Read the model definition and answer for the solid it produces. Units are mm, in the model's axes. A direction names the side the tool comes from. Coordinates: 2 decimals unless noted, no trailing zeros. Loops run counter-clockwise (first coordinate to the right, second up) from the corner with the lowest first, then second, coordinate; pieces in that order, holes last. Notation, with made-up numbers: (-38.75, -12.75) - (-31.75, -12.75) arc R24 ccw to (-31.75, 9.25) - close; hole circle Ø9 at (3.25, 38). An arc over 180 degrees is marked (long way). Use one line per item in the form item = value. Start each with the question number.
1) A cutting plane is placed at B-B (z = -8). Give the vertices of the cut face in (x, y) (3 decimals), and give its area (3 significant figures).
2) A cutting plane is placed at C-C (z = -14.5). Give the vertices of the cut face in (x, y) (3 decimals), and give its area (3 significant figures).
3) A cutting plane is placed at A-A (y = 10.85). Give the vertices of the cut face in (x, z) (3 decimals), and give its area (3 significant figures).
4) Which of the six approach directions +Z, -Z, +X, -X, +Y, -Y give full straight-line access (tool end or side, diameter ignored) to faces 4 (the face through (135, 12, -5.08)), 5 (the face through (135, 3, -19.05)), 6 (the face through (135, 47.117, 10))?
5) A cutting plane is placed at D-D (z = 8). Give the vertices of the cut face in (x, y) (3 decimals), and give its area (3 significant figures).
6) Consider line 1 (Y direction, x = 135.15, z = 10.5); line 2 (Y direction, x = 135, z = -8); line 3 (Y direction, x = 133.9, z = 23.5). Determine where each line is inside the solid, lowest interval first.
7) Each of these flat-tipped pins is pushed along its axis until it touches: P1, Ø1, axis at x = 134.5, y = 84.5, coming from the -Z side; P2, Ø1.6, axis at x = 135.5, y = 18, coming from the +Z side; P3, Ø1, axis at x = 135.5, z = -26.5, coming from the -Y side; P4, Ø5, axis at y = 10.85, z = 14.5, coming from the +X side (3 decimals). Where does it stop, or does it pass through?
8) The mould has two halves that part along Z. Classify faces 1 (the face through (134.96, 64.337, 8.195)), 2 (the face through (135, 43.942, -4)), 3 (the face through (135, 81, -25.4)): released by +Z, released by -Z, zero draft, split by the parting line, or undercut.
from build123d import *

# Parameters (mm, degrees)
SKETCH1_W              = 273.05
SKETCH1_H              = 139.7
BOSS_EXTRUDE1_DEPTH    = 6.35
SKETCH2_W              = 273.05
SKETCH2_H              = 139.7
SKETCH2_W_2            = 266.7
SKETCH2_H_2            = 133.35
BOSS_EXTRUDE2_DEPTH    = 298.45
SKETCH3_W              = 6.35
SKETCH3_H              = 16.933333333
SKETCH3_H_2            = 16.933333334
DOOR_SLOT_DEPTH        = 12.7
DOOR_GUIDE_HOLES_REACH = 362.806
SKETCH4_W              = 6.35
SKETCH4_H              = 15.875
LEVER_HOLES_W          = 9.652
LEVER_HOLES_H          = 6.35
LEVER_HOLES_W_2        = 6.35
CUT_EXTRUDE1_DEPTH     = 363.019620497
CUT_EXTRUDE3_REACH     = 417.137
SKETCH8_R              = 3.175
SKETCH16_W             = 329.651778096
SKETCH16_H             = 315.233565403
CUT_EXTRUDE10_DEPTH    = 363.019620497
LEFT_RIGHT_W           = 9.525
LEFT_RIGHT_H           = 6.35
LEFT_RIGHT_W_2         = 12.7
LEFT_RIGHT_W_3         = 3.175
LEFT_RIGHT_H_2         = 12.7
CUT_EXTRUDE11_DEPTH    = 416.136561869
SKETCH17_W             = 23
SKETCH17_H             = 20.0007988
SKETCH17_W_2           = 10.16
SKETCH17_H_2           = 5.89
SKETCH17_R             = 1.5
CUT_EXTRUDE12_DEPTH    = 313.717353412
CUT_EXTRUDE13_DEPTH    = 313.717353412
CUT_EXTRUDE14_DEPTH    = 106.589636092


with BuildPart() as part:
    # Sketch1 → Boss-Extrude1 (new body)
    with BuildSketch(Plane(origin=(0, 0, 0), x_dir=(1, 0, 0), z_dir=(0, 1, 0))):
        Rectangle(SKETCH1_W, SKETCH1_H)
    extrude(amount=BOSS_EXTRUDE1_DEPTH)

    # Sketch2 → Boss-Extrude2 (add)
    with BuildSketch(Plane(origin=(0, 6.35, 0), x_dir=(1, 0, 0), z_dir=(0, 1, 0))):
        Rectangle(SKETCH2_W, SKETCH2_H)
        Rectangle(SKETCH2_W_2, SKETCH2_H_2, mode=Mode.SUBTRACT)
    extrude(amount=BOSS_EXTRUDE2_DEPTH)

    # Sketch3 → Door Slot (cut)
    with BuildSketch(Plane.XY.offset(69.85)):
        with BuildLine():
            Line((-31.75, 283.21), (-31.75, 6.35))
            Line((-31.75, 6.35), (-25.146, 6.35))
            Line((-25.146, 6.35), (-25.146, 292.354))
            Line((-25.146, 292.354), (-44.704, 292.354))
            Line((-44.704, 292.354), (-44.704, 285.75))
            Line((-44.704, 285.75), (-34.29, 285.75))
            ThreePointArc((-34.29, 285.75), (-32.493948776, 285.006051224), (-31.75, 283.21))
        make_face()
        with Locations((-15.621, 80.433333334)):
            Rectangle(SKETCH3_W, SKETCH3_H)
        with Locations((-15.621, 50.8)):
            Rectangle(SKETCH3_W, SKETCH3_H_2)
        with Locations((-15.621, 21.166666667)):
            Rectangle(SKETCH3_W, SKETCH3_H)
    extrude(amount=-DOOR_SLOT_DEPTH, mode=Mode.SUBTRACT)

    # Sketch4 → Door Guide Holes (cut, up to next)
    with BuildSketch(Plane.XY.offset(-66.675), mode=Mode.PRIVATE) as door_guide_holes_sk1:
        with Locations((-47.879, 284.1625)):
            Rectangle(SKETCH4_W, SKETCH4_H)
    door_guide_holes_tool1 = extrude(door_guide_holes_sk1.sketch, amount=-DOOR_GUIDE_HOLES_REACH, mode=Mode.PRIVATE) & part.part
    # Sketch4 → Door Guide Holes (cut, up to next)
    with BuildSketch(Plane.XY.offset(-66.675), mode=Mode.PRIVATE) as door_guide_holes_sk2:
        with Locations((-47.879, 255.5875)):
            Rectangle(SKETCH4_W, SKETCH4_H)
    door_guide_holes_tool2 = extrude(door_guide_holes_sk2.sketch, amount=-DOOR_GUIDE_HOLES_REACH, mode=Mode.PRIVATE) & part.part
    # Sketch4 → Door Guide Holes (cut, up to next)
    with BuildSketch(Plane.XY.offset(-66.675), mode=Mode.PRIVATE) as door_guide_holes_sk3:
        with Locations((-47.879, 227.0125)):
            Rectangle(SKETCH4_W, SKETCH4_H)
    door_guide_holes_tool3 = extrude(door_guide_holes_sk3.sketch, amount=-DOOR_GUIDE_HOLES_REACH, mode=Mode.PRIVATE) & part.part
    # Sketch4 → Door Guide Holes (cut, up to next)
    with BuildSketch(Plane.XY.offset(-66.675), mode=Mode.PRIVATE) as door_guide_holes_sk4:
        with Locations((-47.879, 198.4375)):
            Rectangle(SKETCH4_W, SKETCH4_H)
    door_guide_holes_tool4 = extrude(door_guide_holes_sk4.sketch, amount=-DOOR_GUIDE_HOLES_REACH, mode=Mode.PRIVATE) & part.part
    # Sketch4 → Door Guide Holes (cut, up to next)
    with BuildSketch(Plane.XY.offset(-66.675), mode=Mode.PRIVATE) as door_guide_holes_sk5:
        with Locations((-47.879, 169.8625)):
            Rectangle(SKETCH4_W, SKETCH4_H)
    door_guide_holes_tool5 = extrude(door_guide_holes_sk5.sketch, amount=-DOOR_GUIDE_HOLES_REACH, mode=Mode.PRIVATE) & part.part
    # Sketch4 → Door Guide Holes (cut, up to next)
    with BuildSketch(Plane.XY.offset(-66.675), mode=Mode.PRIVATE) as door_guide_holes_sk6:
        with Locations((-47.879, 141.2875)):
            Rectangle(SKETCH4_W, SKETCH4_H)
    door_guide_holes_tool6 = extrude(door_guide_holes_sk6.sketch, amount=-DOOR_GUIDE_HOLES_REACH, mode=Mode.PRIVATE) & part.part
    # Sketch4 → Door Guide Holes (cut, up to next)
    with BuildSketch(Plane.XY.offset(-66.675), mode=Mode.PRIVATE) as door_guide_holes_sk7:
        with Locations((-47.879, 112.7125)):
            Rectangle(SKETCH4_W, SKETCH4_H)
    door_guide_holes_tool7 = extrude(door_guide_holes_sk7.sketch, amount=-DOOR_GUIDE_HOLES_REACH, mode=Mode.PRIVATE) & part.part
    # Sketch4 → Door Guide Holes (cut, up to next)
    with BuildSketch(Plane.XY.offset(-66.675), mode=Mode.PRIVATE) as door_guide_holes_sk8:
        with Locations((-47.879, 84.1375)):
            Rectangle(SKETCH4_W, SKETCH4_H)
    door_guide_holes_tool8 = extrude(door_guide_holes_sk8.sketch, amount=-DOOR_GUIDE_HOLES_REACH, mode=Mode.PRIVATE) & part.part
    # Sketch4 → Door Guide Holes (cut, up to next)
    with BuildSketch(Plane.XY.offset(-66.675), mode=Mode.PRIVATE) as door_guide_holes_sk9:
        with Locations((-47.879, 55.5625)):
            Rectangle(SKETCH4_W, SKETCH4_H)
    door_guide_holes_tool9 = extrude(door_guide_holes_sk9.sketch, amount=-DOOR_GUIDE_HOLES_REACH, mode=Mode.PRIVATE) & part.part
    # Sketch4 → Door Guide Holes (cut, up to next)
    with BuildSketch(Plane.XY.offset(-66.675), mode=Mode.PRIVATE) as door_guide_holes_sk10:
        with Locations((-47.879, 26.9875)):
            Rectangle(SKETCH4_W, SKETCH4_H)
    door_guide_holes_tool10 = extrude(door_guide_holes_sk10.sketch, amount=-DOOR_GUIDE_HOLES_REACH, mode=Mode.PRIVATE) & part.part
    door_guide_holes_1 = door_guide_holes_tool1.solids().sort_by_distance((-47.879, 284.1625, -66.675))[0]
    add(door_guide_holes_1, mode=Mode.SUBTRACT)
    door_guide_holes_2 = door_guide_holes_tool2.solids().sort_by_distance((-47.879, 255.5875, -66.675))[0]
    add(door_guide_holes_2, mode=Mode.SUBTRACT)
    door_guide_holes_3 = door_guide_holes_tool3.solids().sort_by_distance((-47.879, 227.0125, -66.675))[0]
    add(door_guide_holes_3, mode=Mode.SUBTRACT)
    door_guide_holes_4 = door_guide_holes_tool4.solids().sort_by_distance((-47.879, 198.4375, -66.675))[0]
    add(door_guide_holes_4, mode=Mode.SUBTRACT)
    door_guide_holes_5 = door_guide_holes_tool5.solids().sort_by_distance((-47.879, 169.8625, -66.675))[0]
    add(door_guide_holes_5, mode=Mode.SUBTRACT)
    door_guide_holes_6 = door_guide_holes_tool6.solids().sort_by_distance((-47.879, 141.2875, -66.675))[0]
    add(door_guide_holes_6, mode=Mode.SUBTRACT)
    door_guide_holes_7 = door_guide_holes_tool7.solids().sort_by_distance((-47.879, 112.7125, -66.675))[0]
    add(door_guide_holes_7, mode=Mode.SUBTRACT)
    door_guide_holes_8 = door_guide_holes_tool8.solids().sort_by_distance((-47.879, 84.1375, -66.675))[0]
    add(door_guide_holes_8, mode=Mode.SUBTRACT)
    door_guide_holes_9 = door_guide_holes_tool9.solids().sort_by_distance((-47.879, 55.5625, -66.675))[0]
    add(door_guide_holes_9, mode=Mode.SUBTRACT)
    door_guide_holes_10 = door_guide_holes_tool10.solids().sort_by_distance((-47.879, 26.9875, -66.675))[0]
    add(door_guide_holes_10, mode=Mode.SUBTRACT)
    door_guide_holes = door_guide_holes_1 + door_guide_holes_2 + door_guide_holes_3 + door_guide_holes_4 + door_guide_holes_5 + door_guide_holes_6 + door_guide_holes_7 + door_guide_holes_8 + door_guide_holes_9 + door_guide_holes_10  # Door Guide Holes as one shape, for the pattern or mirror that repeats it

    # Mirror1: Door Guide Holes across plane
    add(door_guide_holes.mirror(Plane.ZY.offset(34.925)), mode=Mode.SUBTRACT)

    # Lever Holes → Cut-Extrude1 (cut, through all)
    with BuildSketch(Plane.XY.offset(69.85)):
        with Locations((54.102, 28.575)):
            Rectangle(LEVER_HOLES_W, LEVER_HOLES_H)
        with Locations((39.3065, 15.875)):
            Rectangle(LEVER_HOLES_W_2, LEVER_HOLES_H)
        with Locations((68.8975, 15.875)):
            Rectangle(LEVER_HOLES_W_2, LEVER_HOLES_H)
    extrude(amount=-CUT_EXTRUDE1_DEPTH, mode=Mode.SUBTRACT)

    # Sketch8 → Cut-Extrude3 (cut, up to next)
    with BuildSketch(Plane.ZY.offset(136.525), mode=Mode.PRIVATE) as cut_extrude3_sk1:
        with Locations((0, 19.05)):
            Circle(SKETCH8_R)
    cut_extrude3_tool1 = extrude(cut_extrude3_sk1.sketch, amount=-CUT_EXTRUDE3_REACH, mode=Mode.PRIVATE) & part.part
    add(cut_extrude3_tool1.solids().sort_by_distance((-136.525, 19.05, 0))[0], mode=Mode.SUBTRACT)

    # Sketch16 → Cut-Extrude10 (cut, through all)
    with BuildSketch(Plane.XY.offset(69.85)):
        with Locations((-31.475889048, 147.183217299)):
            Rectangle(SKETCH16_W, SKETCH16_H)
    extrude(amount=-CUT_EXTRUDE10_DEPTH, mode=Mode.SUBTRACT)

    # Left/Right → Cut-Extrude11 (cut, through all)
    with BuildSketch(Plane.ZY.offset(136.525)):
        with Locations((61.9125, 3.175)):
            Rectangle(LEFT_RIGHT_W, LEFT_RIGHT_H)
        with Locations((38.1, 3.175)):
            Rectangle(LEFT_RIGHT_W_2, LEFT_RIGHT_H)
        with Locations((68.2625, 19.05)):
            Rectangle(LEFT_RIGHT_W_3, LEFT_RIGHT_H_2)
        with Locations((12.7, 3.175)):
            Rectangle(LEFT_RIGHT_W_2, LEFT_RIGHT_H)
        with Locations((68.2625, 44.45)):
            Rectangle(LEFT_RIGHT_W_3, LEFT_RIGHT_H_2)
        with Locations((-12.7, 3.175)):
            Rectangle(LEFT_RIGHT_W_2, LEFT_RIGHT_H)
        with Locations((68.2625, 69.85)):
            Rectangle(LEFT_RIGHT_W_3, LEFT_RIGHT_H_2)
        with Locations((-38.1, 3.175)):
            Rectangle(LEFT_RIGHT_W_2, LEFT_RIGHT_H)
        with Locations((68.2625, 95.25)):
            Rectangle(LEFT_RIGHT_W_3, LEFT_RIGHT_H_2)
        with Locations((-61.9125, 3.175)):
            Rectangle(LEFT_RIGHT_W, LEFT_RIGHT_H)
        with Locations((68.2625, 120.65)):
            Rectangle(LEFT_RIGHT_W_3, LEFT_RIGHT_H_2)
        with Locations((-68.2625, 19.05)):
            Rectangle(LEFT_RIGHT_W_3, LEFT_RIGHT_H_2)
        with Locations((68.2625, 146.05)):
            Rectangle(LEFT_RIGHT_W_3, LEFT_RIGHT_H_2)
        with Locations((-68.2625, 44.45)):
            Rectangle(LEFT_RIGHT_W_3, LEFT_RIGHT_H_2)
        with Locations((68.2625, 171.45)):
            Rectangle(LEFT_RIGHT_W_3, LEFT_RIGHT_H_2)
        with Locations((-68.2625, 69.85)):
            Rectangle(LEFT_RIGHT_W_3, LEFT_RIGHT_H_2)
        with Locations((68.2625, 196.85)):
            Rectangle(LEFT_RIGHT_W_3, LEFT_RIGHT_H_2)
        with Locations((-68.2625, 95.25)):
            Rectangle(LEFT_RIGHT_W_3, LEFT_RIGHT_H_2)
        with Locations((68.2625, 222.25)):
            Rectangle(LEFT_RIGHT_W_3, LEFT_RIGHT_H_2)
        with Locations((-68.2625, 120.65)):
            Rectangle(LEFT_RIGHT_W_3, LEFT_RIGHT_H_2)
        with Locations((68.2625, 247.65)):
            Rectangle(LEFT_RIGHT_W_3, LEFT_RIGHT_H_2)
        with Locations((-68.2625, 146.05)):
            Rectangle(LEFT_RIGHT_W_3, LEFT_RIGHT_H_2)
        with Locations((68.2625, 273.05)):
            Rectangle(LEFT_RIGHT_W_3, LEFT_RIGHT_H_2)
        with Locations((-68.2625, 171.45)):
            Rectangle(LEFT_RIGHT_W_3, LEFT_RIGHT_H_2)
        with Locations((68.2625, 298.45)):
            Rectangle(LEFT_RIGHT_W_3, LEFT_RIGHT_H_2)
        with Locations((-68.2625, 196.85)):
            Rectangle(LEFT_RIGHT_W_3, LEFT_RIGHT_H_2)
        with Locations((-68.2625, 222.25)):
            Rectangle(LEFT_RIGHT_W_3, LEFT_RIGHT_H_2)
        with Locations((-68.2625, 247.65)):
            Rectangle(LEFT_RIGHT_W_3, LEFT_RIGHT_H_2)
        with Locations((-68.2625, 273.05)):
            Rectangle(LEFT_RIGHT_W_3, LEFT_RIGHT_H_2)
        with Locations((-68.2625, 298.45)):
            Rectangle(LEFT_RIGHT_W_3, LEFT_RIGHT_H_2)
    extrude(amount=-CUT_EXTRUDE11_DEPTH, mode=Mode.SUBTRACT)

    # Sketch17 → Cut-Extrude12 (cut, through all)
    with BuildSketch(Plane(origin=(136.525, 0, 0), x_dir=(0, 0, -1), z_dir=(1, 0, 0))):
        with Locations((0, 25.2403994)):
            Rectangle(SKETCH17_W, SKETCH17_H)
        with Locations((0, 12.295)):
            Rectangle(SKETCH17_W_2, SKETCH17_H_2)
        with Locations((14.5, 10.85)):
            Circle(SKETCH17_R)
        with Locations((-14.5, 10.85)):
            Circle(SKETCH17_R)
        with Locations((-8, 62.8499886)):
            Circle(SKETCH17_R)
        with Locations((8, 62.8499886)):
            Circle(SKETCH17_R)
    extrude(amount=-CUT_EXTRUDE12_DEPTH, mode=Mode.SUBTRACT)

    # Sketch18 → Cut-Extrude13 (cut, through all)
    with BuildSketch(Plane(origin=(136.525, 0, 0), x_dir=(0, 0, -1), z_dir=(1, 0, 0))):
        Polygon((-69.85, 304.8), (-69.85, 0), (-25.4, 0), (-25.4, 53.467), (-28.575, 53.467), (-28.575, 59.817), (-25.4, 59.817), (-25.4, 101.6), (25.4, 101.6), (25.4, 59.817), (28.575, 59.817), (28.575, 53.467), (25.4, 53.467), (25.4, 0), (69.85, 0), (69.85, 304.8), align=None)
    extrude(amount=-CUT_EXTRUDE13_DEPTH, mode=Mode.SUBTRACT)

    # Sketch19 → Cut-Extrude14 (cut, through all)
    with BuildSketch(Plane.ZY.offset(-133.35)):
        Polygon((25.4, 47.117), (-6.35, 47.117), (-6.35, 43.942), (-1.5875, 43.942), (-1.5875, 37.592), (4.8895, 37.592), (4.8895, 43.942), (25.4, 43.942), align=None)
    extrude(amount=-CUT_EXTRUDE14_DEPTH, mode=Mode.SUBTRACT)


solid = part.part
Found:
q1.outline = (133.35, 6.35) - (136.525, 6.35) - (136.525, 15.24) - (133.35, 15.24) - close; (133.35, 35.241) - (136.525, 35.241) - (136.525, 61.35) - (133.35, 61.35) - close; (133.35, 64.35) - (136.525, 64.35) - (136.525, 101.6) - (133.35, 101.6) - close
q1.area = 229 mm^2
q2.outline = (133.35, 6.35) - (136.525, 6.35) - (136.525, 9.35) - (133.35, 9.35) - close; (133.35, 12.35) - (136.525, 12.35) - (136.525, 101.6) - (133.35, 101.6) - close
q2.area = 293 mm^2
q3.outline = (133.35, -25.4) - (136.525, -25.4) - (136.525, -16) - (133.35, -16) - close; (133.35, -13) - (136.525, -13) - (136.525, -5.08) - (133.35, -5.08) - close; (133.35, 5.08) - (136.525, 5.08) - (136.525, 13) - (133.35, 13) - close; (133.35, 16) - (136.525, 16) - (136.525, 25.4) - (133.35, 25.4) - close
q3.area = 110 mm^2
q4.face_4 = +X, -X
q4.face_5 = +X, -X, -Y
q4.face_6 = +Z, +X, -X
q5.outline = (133.35, 6.35) - (136.525, 6.35) - (136.525, 15.24) - (133.35, 15.24) - close; (133.35, 35.241) - (136.525, 35.241) - (136.525, 43.942) - (133.35, 43.942) - close; (133.35, 47.117) - (136.525, 47.117) - (136.525, 61.35) - (133.35, 61.35) - close; (133.35, 64.35) - (136.525, 64.35) - (136.525, 101.6) - (133.35, 101.6) - close
q5.area = 219 mm^2
q6.line_1 = 6.35 to 15.24, 35.24 to 43.94, 47.12 to 101.6
q6.line_2 = 6.35 to 15.24, 35.24 to 61.35, 64.35 to 101.6
q6.line_3 = 0 to 43.94, 47.12 to 101.6
q7.P1 = -25.4
q7.P2 = 25.4
q7.P3 = 53.47
q7.P4 = 136.525
q8.face_1 = undercut
q8.face_2 = zero draft
q8.face_3 = released by -Z
